Geometry: see drawing. Coordinates: mm, zero at the bounding-box minimum. Round coordinates to 2 decimals unless told otherwise and drop trailing zeros. Loops run counter-clockwise (first coordinate to the right, second up) from the corner with the lowest first, then second, coordinate; pieces in that order, holes last. Notation, with made-up numbers: (18, -26) - (35, -26) arc R24 ccw to (35, 10) - close; hole circle Ø1 at (13, -30). An arc over 180 degrees is marked (long way). Use CSV: the item, a comma, the result in double quotes. Start each with the question number.
1. Pin query (flat end, axial travel): P1, Ø1.5, axis at y = 183.5, z = 1.5, coming from the +X side; P2, Ø2.5, axis at y = 2.5, z = 3.5, coming from the -X side; P3, Ø1.5, axis at x = 173.5, z = 1.5, coming from the +Y side. Return the tip coordinate at first contact, or that it passes through.
2. Cut plane A-A (x = 125). Return loops of the section in (y, z), and give its area (3 significant figures).
3. Material intervals for probe 1 along Y at (x, z) = (125, 2.6); probe 2 along Y at (x, z) = (133.5, 3.25); probe 3 along X at (y, z) = (62.5, 4.5), sorted ascending. Write a range as from..to.
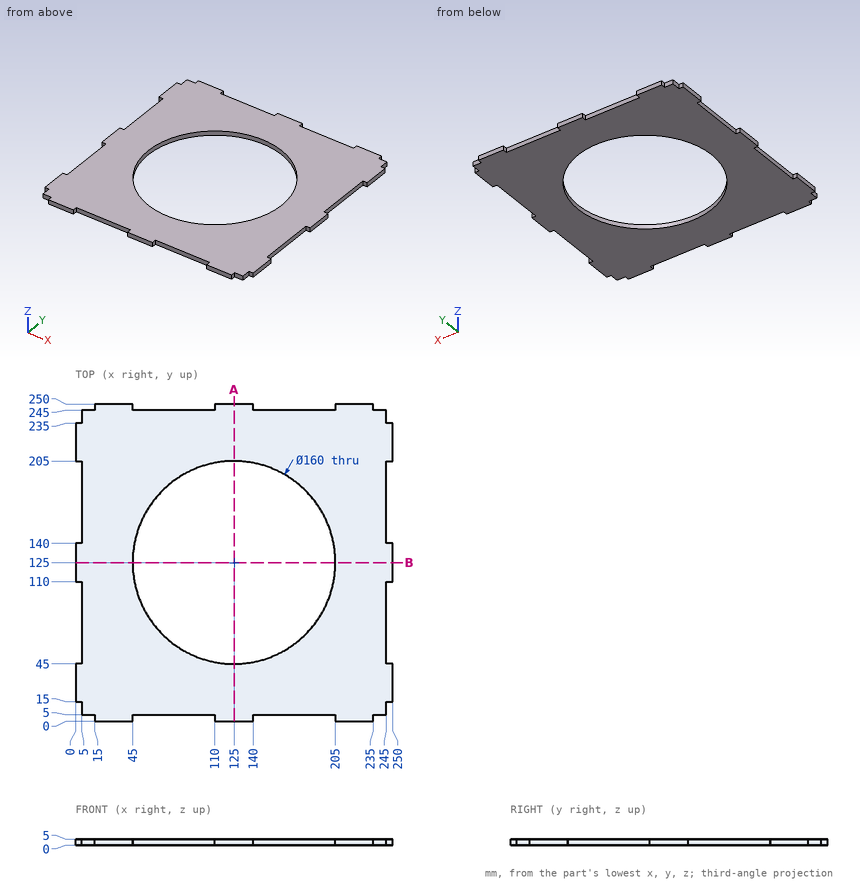
Established:
1,P1,"stops at x = 245"
1,P2,"stops at x = 15"
1,P3,"stops at y = 245"
2,outline,"(0, 0) - (45, 0) - (45, 5) - (0, 5) - close; (205, 0) - (250, 0) - (250, 5) - (205, 5) - close"
2,area,"450 mm2"
3,probe 1,"y = 0..45, 205..250"
3,probe 2,"y = 0..45.45, 204.55..250"
3,probe 3,"x = 5..75.06, 174.94..245"
